Input: dimensioned drawing with shaded views. Units: mm. Origin: part minimum x, y, z. Give positions to 0.01 mm unless a question says otherwise; leave off trailing zeros. Write each loop counter-clockwise with the first axis right and the second up, starting at its lowest first coordinate (ties: lowest second). Pieces come first, ordered by that corner, then holes.
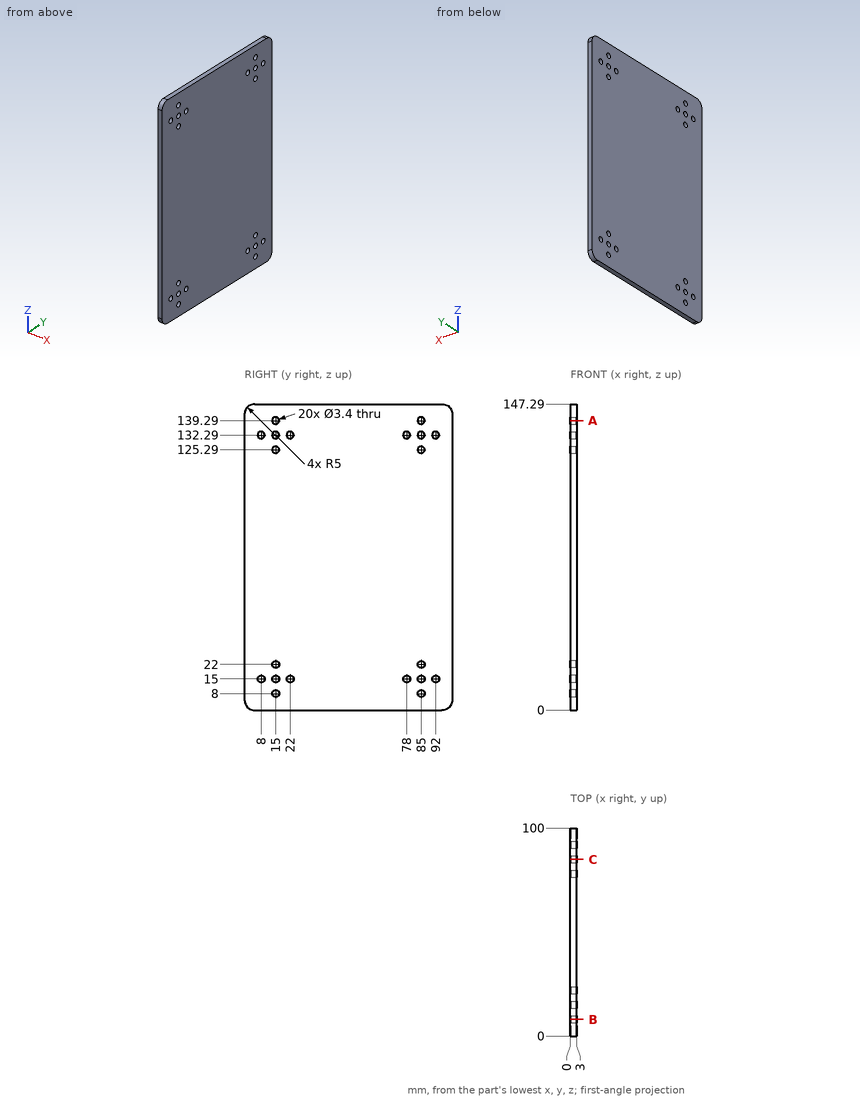
1. Cut plane C-C, the plane y = 85. Return the cut outline in (x, z).
2. Cut plane B-B, the plane y = 8. Return the cut outline in (x, z), then the cut area to 3 significant figures.
3. Cut plane A-A, the plane z = 139.29. Return the cut outline in (x, y).
4. Line query: L1, parallel to Y at x = 1.45, z = 8; L2, parallel to Y at x = 1.85, z = 140. Output: solid intervals per line, ascending.
Response values:
1. outline: (0, 0) - (3, 0) - (3, 6.3) - (0, 6.3) - close; (0, 9.7) - (3, 9.7) - (3, 13.3) - (0, 13.3) - close; (0, 16.7) - (3, 16.7) - (3, 20.3) - (0, 20.3) - close; (0, 23.7) - (3, 23.7) - (3, 123.59) - (0, 123.59) - close; (0, 126.99) - (3, 126.99) - (3, 130.59) - (0, 130.59) - close; (0, 133.99) - (3, 133.99) - (3, 137.59) - (0, 137.59) - close; (0, 140.99) - (3, 140.99) - (3, 147.29) - (0, 147.29) - close
2. outline: (0, 0) - (3, 0) - (3, 13.3) - (0, 13.3) - close; (0, 16.7) - (3, 16.7) - (3, 130.59) - (0, 130.59) - close; (0, 133.99) - (3, 133.99) - (3, 147.29) - (0, 147.29) - close
2. area: 421 mm2
3. outline: (0, 0) - (3, 0) - (3, 13.3) - (0, 13.3) - close; (0, 16.7) - (3, 16.7) - (3, 83.3) - (0, 83.3) - close; (0, 86.7) - (3, 86.7) - (3, 100) - (0, 100) - close
4. L1: y = 0 to 13.3, 16.7 to 83.3, 86.7 to 100
4. L2: y = 0 to 13.46, 16.54 to 83.46, 86.54 to 100
